Source: CAD feature listing. Evaluate the final solid. Frame: model axes, mm. Face numbers are marked on the shaded views. A direction names the side the tool comes from. Round coordinates to 2 decimals unless told otherwise and drop trailing zeros. Loops run counter-clockwise (first coordinate to the right, second up) from the corner with the lowest first, then second, coordinate; pieces in that order, holes last.
(1) Set-up query: the marked faces 1 and 2. Return all of +Z, -Z, +X, -X, +Y, -Y with unobstructed straight access to the full face (end or side cutting, diameter ignored); none if empty.
(2) Material intervals for probe 1 along X at (y, z) = (-5.5, -10); probe 2 along Z at (x, y) = (5, 0); probe 3 along Y at (x, z) = (0.5, -3.5), sorted ascending.
(3) First-contact query: pin 1 Ø1.5 at (y, z) = (14, 5.5) entering from +X; pin 2 Ø2 at (x, y) = (2.5, -13.5) entering from +Z; pin 3 Ø3 at (x, y) = (7, -0.5) entering from +Z; pin 4 Ø1.9 at (y, z) = (0, 0) entering from -X. Flat tips, straight axial feed; report the tip coordinate or a pass-through.
(4) Section C-C, the plane x = 5.25. Return the cut outline in (y, z) (1 decimal), plus the area to 3 significant figures.
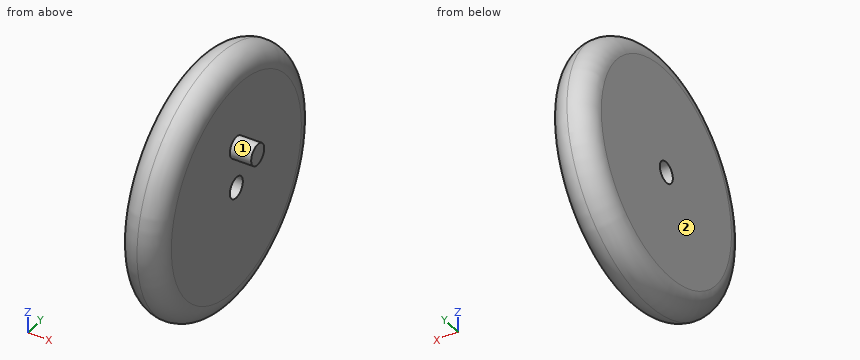
```python
from build123d import *

# Parameters (mm, degrees)
F0_R     = 19.05
F3_DEPTH = 6.35
F2_R     = 1.5875
F4_DEPTH = 6.35
F5_R     = 3.175
F6_R     = 3.17499
F7_R     = 1.5875
F8_DEPTH = 3.175


# Not quite as in the source:
# - a fillet or chamfer is up to 0.001 mm smaller than in the source, because OpenCascade refuses the exact size


with BuildPart() as f3:
    # F0 (on Right) → F3 (new body)
    with BuildSketch(Plane.YZ):
        Circle(F0_R)
    extrude(amount=F3_DEPTH)

    # F2 (on face) → F4 (cut)
    with BuildSketch(Plane.YZ):
        Circle(F2_R)
    extrude(amount=F4_DEPTH, mode=Mode.SUBTRACT)

    # F5
    f5_edges = [f3.edges().sort_by_distance(p)[0] for p in [
        (0, -19.05, 0),
    ]]
    fillet(f5_edges, radius=F5_R)

    # F6 (radius 3.175 in the source; OpenCascade refuses exactly that, so slightly less here)
    f6_edges = [f3.edges().sort_by_distance(p)[0] for p in [
        (6.35, -19.05, 0),
    ]]
    fillet(f6_edges, radius=F6_R)

    # F7 (on face) → F8 (join)
    with BuildSketch(Plane.YZ.offset(6.35)):
        with Locations((0, 6.35)):
            Circle(F7_R)
    extrude(amount=F8_DEPTH)


solid = f3.part
```
Output values:
1. face 1: +X
1. face 2: +Z, -Z, -X, +Y, -Y
2. probe 1: x = 0 to 6.35
2. probe 2: z = -18.47 to -1.59, 1.59 to 18.47
2. probe 3: y = -17.23 to 17.23
3. pin 1: stops at x = 6.35
3. pin 2: stops at z = 14.31
3. pin 3: stops at z = 18.03
3. pin 4: passes through
4. outline: circle Ø36.6 at (0, 0); hole circle Ø3.2 at (0, 0)
4. area: 1,040 mm2
